Design review of the part built by this model. Coordinates are the model's own, in mm. Face numbers are marked on the shaded views. A direction names the side the tool comes from. Coordinates: 2 decimals unless noted, no trailing zeros. Order: outer loops, then holes, each group sorted by start corner. A loop starts at its lowest first (then second) coordinate and runs counter-clockwise, first axis right, second up. Notation, with made-up numbers: M 39,-25 L 85,-25 A32 ccw 85,4 Z; hole C -20,4 d8. An arc over 180 degrees is marked long. Answer as a JSON object with one key per item and string values.
from build123d import *

# Parameters (mm, degrees)
SKETCH1_R               = 9
BOSS_EXTRUDE1_DEPTH     = 24
SKETCH2_R               = 8
BOSS_EXTRUDE2_DEPTH     = 10
SKETCH3_R               = 6
BOSS_EXTRUDE3_DEPTH     = 10
SKETCH4_R               = 8
BOSS_EXTRUDE4_DEPTH     = 82
SKETCH5_R               = 6
BOSS_EXTRUDE5_DEPTH     = 9
SKETCH6_R               = 4
BOSS_EXTRUDE6_DEPTH     = 6
SKETCH7_R               = 6
BOSS_EXTRUDE7_DEPTH     = 7
SKETCH8_R               = 3
CUT_EXTRUDE1_DEPTH      = 10
CUT_EXTRUDE1_DEPTH_BACK = 10


with BuildPart() as part:
    # Sketch1 → Boss-Extrude1 (new body)
    with BuildSketch(Plane(origin=(0, 0, 0), x_dir=(1, 0, 0), z_dir=(0, 1, 0))):
        Circle(SKETCH1_R)
    extrude(amount=BOSS_EXTRUDE1_DEPTH)

    # Sketch2 → Boss-Extrude2 (add)
    with BuildSketch(Plane(origin=(0, 24, 0), x_dir=(1, 0, 0), z_dir=(0, 1, 0))):
        Circle(SKETCH2_R)
    extrude(amount=BOSS_EXTRUDE2_DEPTH)

    # Sketch3 → Boss-Extrude3 (add)
    with BuildSketch(Plane(origin=(0, 34, 0), x_dir=(1, 0, 0), z_dir=(0, 1, 0))):
        Circle(SKETCH3_R)
    extrude(amount=BOSS_EXTRUDE3_DEPTH)

    # Sketch4 → Boss-Extrude4 (add)
    with BuildSketch(Plane(origin=(0, 44, 0), x_dir=(1, 0, 0), z_dir=(0, 1, 0))):
        Circle(SKETCH4_R)
    extrude(amount=BOSS_EXTRUDE4_DEPTH)

    # Sketch5 → Boss-Extrude5 (add)
    with BuildSketch(Plane(origin=(0, 126, 0), x_dir=(1, 0, 0), z_dir=(0, 1, 0))):
        Circle(SKETCH5_R)
    extrude(amount=BOSS_EXTRUDE5_DEPTH)

    # Sketch6 → Boss-Extrude6 (add)
    with BuildSketch(Plane(origin=(0, 135, 0), x_dir=(1, 0, 0), z_dir=(0, 1, 0))):
        Circle(SKETCH6_R)
    extrude(amount=BOSS_EXTRUDE6_DEPTH)

    # Sketch7 → Boss-Extrude7 (add)
    with BuildSketch(Plane(origin=(0, 141, 0), x_dir=(1, 0, 0), z_dir=(0, 1, 0))):
        Circle(SKETCH7_R)
    extrude(amount=BOSS_EXTRUDE7_DEPTH)

    # Sketch8 → Cut-Extrude1 (cut, two sides)
    with BuildSketch(Plane.XY) as cut_extrude1_sk:
        with Locations((0, 12)):
            Circle(SKETCH8_R)
    extrude(amount=CUT_EXTRUDE1_DEPTH, mode=Mode.SUBTRACT)
    extrude(cut_extrude1_sk.sketch, amount=-CUT_EXTRUDE1_DEPTH_BACK, mode=Mode.SUBTRACT)


solid = part.part
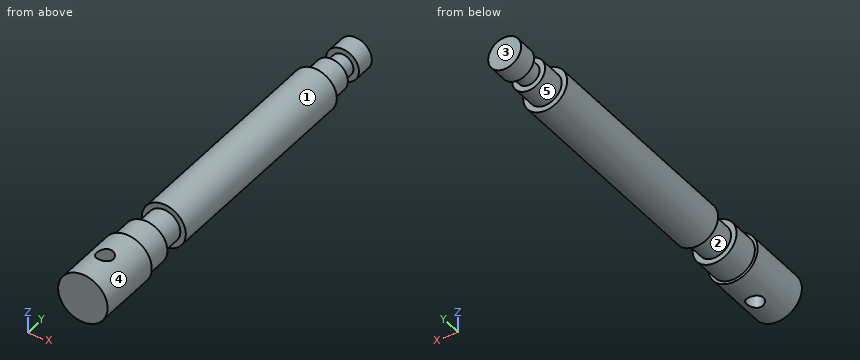
1) Add section B-B (y = 93). State the section outline as (x, z) points, and give its area (3 significant figures).
Taken from the geometry:
{"outline": "C 0,0 d16", "area": "201 mm2"}
2) To check wall thickness, follow L1, parallel to Y at x = 0, z = -4.25; L2, parallel to Y at x = 0, z = -7; L3, parallel to Y at x = 0, z = -2.5. State the ranges of each line that lie inside material, in increasing order.
Taken from the geometry:
{"L1": "y = 0 to 9, 15 to 135, 141 to 148", "L2": "y = 0 to 9, 15 to 34, 44 to 126", "L3": "y = 0 to 9, 15 to 148"}
3) Add section C-C (y = 12). State the section outline as (x, z) points.
Taken from the geometry:
{"outline": "M -3,-8.49 L -3,8.49 A9 ccw Z; M 3,-8.49 A9 ccw 3,8.49 Z"}
4) Tool access review of the marked faces 4 and 5: name each direction out of +Z, -Z, +X, -X, +Y, -Y from which nothing blocks a thin tool from reaching the whole face with its end or side.
Taken from the geometry:
{"face 4": "+Y, -Y", "face 5": "+Y"}
5) Mouldability with a two-part tool opening along Y and no side actions: class the marked faces 1, 2 and 3 as released by +Y, released by -Y, zero draft, split by the parting line, or undercut.
Taken from the geometry:
{"face 1": "zero draft", "face 2": "undercut", "face 3": "released by +Y"}
6) Insertion check: pin 1 Ø3 at (x, z) = (7, 6.5) entering from +Y; pin 2 Ø5.5 at (x, y) = (0, 12) entering from -Z; pin 3 Ø6 at (x, y) = (4.5, 91.5) entering from -Z; pin 4 Ø5 at (y, z) = (53.5, 3.5) entering from +X. Each pin has a flat end and moves straight along its axis. Give the tip position at first contact, or say it passes through.
Taken from the geometry:
{"pin 1": "stops at y = 24", "pin 2": "passes through", "pin 3": "stops at z = -7.86", "pin 4": "stops at x = 7.94"}
